Can you work these out from the model? Positions are in its coordinate system, mm. A direction names the side the tool comes from. Round coordinates to 2 decimals unless told otherwise and drop trailing zeros. Order: outer loops, then holes, each group sorted by start corner. A loop starts at its lowest first (then second) coordinate and runs counter-clockwise, first axis right, second up. Notation, with made-up numbers: M 62.5,-3.5 L 98.5,-3.5 A35 ccw 98.5,34.5 Z; hole C -39,21 d3. An arc over 180 degrees is marked long. One line per question, with ' | ' between items.
Autodesk Inventor part; units mm, degrees
ref_plane "Work Plane2" through (30.0013, 0, 7.4992) normal (0, 0, -1) x (-1, 0, 0)
ref_plane "YZ Plane" through (0, 0, 0) normal (1, 0, 0) x (0, 1, 0)
ref_plane "XZ Plane" through (0, 0, 0) normal (0, 1, 0) x (-1, 0, 0)
sketch "Sketch1" plane through (0, 0, 0) normal (0, 1, 0) x (-1, 0, 0)
  line L0 (40, 90) -> (-40, 90)
  line L1 (-40, 90) -> (-40, -81.7795)
  line L2 (40, -41.5685) -> (40, 90)
  line L3 (40, 90) -> (-40, -90) construction
  line L4 (-40, 90) -> (40, -90) construction
  circle A0 centre (-0.0013, 54.9992) radius 5.1
  line L5 (23.4987, -16.5008) -> (-23.5013, -16.5008) construction
  line L6 (-23.5013, -16.5008) -> (-23.5013, -63.5008) construction
  line L7 (-23.5013, -63.5008) -> (23.4987, -63.5008) construction
  line L8 (23.4987, -63.5008) -> (23.4987, -16.5008) construction
  line L9 (23.4987, -16.5008) -> (-23.5013, -63.5008) construction
  line L10 (-23.5013, -16.5008) -> (23.4987, -63.5008) construction
  circle A1 centre (23.4987, -16.5008) radius 2.75
  circle A2 centre (23.4987, -63.5008) radius 2.75
  circle A3 centre (-23.5013, -16.5008) radius 2.75
  circle A4 centre (-23.5013, -63.5008) radius 2.75
  line L11 (-0.0013, -90.0008) -> (-0.0013, -80) construction
  line L12 (19.9987, -11.0008) -> (-20.0013, -11.0008) construction
  line L13 (-20.0013, -11.0008) -> (-20.0013, -69.0008) construction
  line L14 (-20.0013, -69.0008) -> (19.9987, -69.0008) construction
  line L15 (19.9987, -69.0008) -> (19.9987, -11.0008) construction
  line L16 (19.9987, -11.0008) -> (-20.0013, -69.0008) construction
  line L17 (-20.0013, -11.0008) -> (19.9987, -69.0008) construction
  line L18 (-29.0013, -60.0008) -> (28.9987, -60.0008) construction
  line L19 (28.9987, -60.0008) -> (28.9987, -20.0008) construction
  line L20 (28.9987, -20.0008) -> (-29.0013, -20.0008) construction
  line L21 (-29.0013, -20.0008) -> (-29.0013, -60.0008)
  line L22 (-29.0013, -60.0008) -> (28.9987, -20.0008) construction
  line L23 (28.9987, -60.0008) -> (-29.0013, -20.0008) construction
  line L24 (-0.0013, 54.9992) -> (102.5291, -47.5313) construction
  line L25 (-0.0013, 54.9992) -> (144.9987, 54.9992) construction
  line L26 (28.2843, 83.2843) -> (-28.2843, 26.7157) construction
  line L27 (-28.2843, 26.7157) -> (74.2462, -75.8148) construction
  line L28 (74.2462, -75.8148) -> (130.8148, -19.2462) construction
  line L29 (130.8148, -19.2462) -> (28.2843, 83.2843) construction
  line L30 (28.2843, 83.2843) -> (74.2462, -75.8148) construction
  line L31 (-28.2843, 26.7157) -> (130.8148, -19.2462) construction
  line L32 (74.2462, -75.8148) -> (14.1407, -135.9202)
  line L33 (14.1407, -135.9202) -> (-0.0014, -121.7781)
  line L34 (-0.0014, -121.7781) -> (-31.7795, -90)
  line L35 (74.2462, -75.8148) -> (40, -41.5685)
  line L36 (-31.7795, -90) -> (-40, -81.7795)
  line L37 (44.1935, -105.8675) -> (37.1224, -98.7964)
  line L38 (37.1224, -98.7964) -> (52.1488, -83.7701) construction
  line L39 (37.1224, -98.7964) -> (22.096, -113.8228) construction
  circle A5 centre (52.1488, -83.7701) radius 2.75
  circle A6 centre (22.096, -113.8228) radius 2.75
  line L40 (-0.0013, 54.9992) -> (-0.0013, -40.0008)
  circle A7 centre (-0.0013, -40.0008) radius 22.5
  point P0 (0, 0)
  point P1 (51.2639, 3.7339)
  dimension "d0" = 80
  dimension "d1" = 180
  dimension "d3" = 10.2
  dimension "d5" = 47
  dimension "d6" = 47
  dimension "d7" = 5.5
  dimension "d8" = 5.5
  dimension "d9" = 5.5
  dimension "d10" = 5.5
  dimension "d12" = 40
  dimension "d13" = 58
  dimension "d14" = 58
  dimension "d15" = 40
  dimension "d27" = 45
  dimension "d28" = 145
  dimension "d29" = 80
  dimension "d30" = 145
  dimension "d31" = 85.002
  dimension "d32" = 20
  dimension "d33" = 10
  dimension "d35" = 21.2505
  dimension "d36" = 21.2505
  dimension "d37" = 5.5
  dimension "d38" = 5.5
  dimension "d53" = 95
  dimension "d54" = 45
extrude "Plate3" add sketch "Sketch1" along normal blind 6
fillet "Fillet6" radius 5 4 edges at (-40, 3, -41.5685) (-74.2462, 3, -75.8148) (-14.1407, 3, -135.9202) (40, 3, -81.7795)
fillet "Fillet7" radius 40 2 edges at (40, 3, 90) (-40, 3, 90)
sketch "Sketch2" plane through (0, 0, 0) normal (0, -1, 0) x (1, 0, 0)
  circle A0 centre (0.0013, 54.9992) radius 5.1
  line L0 (0.0013, 54.9992) -> (0.0013, -40.0008) construction
  line L1 (0.0013, 7.4992) -> (55.0013, 7.4992) construction
  line L2 (0.0013, 7.4992) -> (-54.9987, 7.4992) construction
  line L3 (-29.9987, 7.4992) -> (30.0013, 7.4992) construction
  line L4 (-29.9987, 4.7492) -> (30.0013, 4.7492)
  line L5 (30.0013, 10.2492) -> (-29.9987, 10.2492)
  arc A1 (-29.9987, 10.2492) -> (-29.9987, 4.7492) centre (-29.9987, 7.4992) ccw
  arc A2 (30.0013, 4.7492) -> (30.0013, 10.2492) centre (30.0013, 7.4992) ccw
  point P0 (0, 0)
  dimension "d43" = 95
  dimension "d44" = 55
  dimension "d45" = 55
  dimension "d46" = 30
  dimension "d47" = 5.5
extrude "Extrusion1" cut sketch "Sketch2" against normal blind 10 contours A1 L5 A2 L4
ref_plane "Work Plane2" through (30.0013, 0, 7.4992) normal (0, 0, -1) x (-1, 0, 0)
equation "\"d39\" = Thickness"
equation "\"BendRadius\" = Thickness"
equation "\"BendReliefWidth\" = Thickness"
equation "\"BendReliefDepth\" = 0.5 * Thickness"
equation "\"CornerReliefSize\" = 4 * Thickness"
equation "\"MinimumRemnant\" = 2 * Thickness"
equation "\"TransitionRadius\" = BendRadius"
equation "\"JacobiRadiusSize\" = BendRadius"
equation "\"GapSize\" = Thickness"
properties part number "NEMA23MountPlatev2" material "Aluminum 6061"
(1) Please list where these lines run through material, in increasing order: probe 1 along Z at (x, y) = (-9, 3.2); probe 2 along Z at (x, y) = (4, 4.05); probe 3 along Z at (x, y) = (23, 2.7). Write a range as [from, to].
Final values:
probe 1: [-130.78, -60.62], [-19.38, 4.75], [10.25, 88.97] | probe 2: [-117.78, -62.14], [-17.86, 4.75], [10.25, 51.83], [58.16, 89.8] | probe 3: [-98.78, -66.2], [-60.8, -19.2], [-13.8, 4.75], [10.25, 82.73]
(2) If we section it at D-D on z = 2: Please give me the cut outline in (x, y).
Final values:
outline: M -40,0 L 40,0 L 40,6 L -40,6 Z
(3) Will these pins go through, and if not, where does the flat tip stop? pin 1 Ø2 at (x, y) = (15.5, 3) entering from +Z; pin 2 Ø2 at (x, y) = (-39, 3) entering from -Z; pin 3 Ø1.8 at (x, y) = (12.5, 1.5) entering from +Z.
Final values:
pin 1: z = 87.28 | pin 2: z = -112.06 | pin 3: z = 88.28
(4) If we section it at B-B on y = 1.6: State how many separate pieces and enclosed holes the cut face has, plus the area to 3 significant figures.
Final values:
separate pieces: 1 | enclosed holes: 9 | area: 14,600 mm^2
(5) Thinking about a two-plate mould opening in X: for faces 1 (the cylindrical face through (4.879, 2.958, -18.036)), 2 (the cylindrical face through (-72.175, 3.042, -75.87)), 3 (the flat face through (13.62, 2.96, -108.16)), which applies, released by +X, released by -X, zero draft, split by the parting line, or undercut?
Final values:
face 1: undercut | face 2: released by -X | face 3: released by +X
(6) On a 3-axis mill with a long thin cutter (end or side, diameter ignored), from which of +Z, -Z, +X, -X, +Y, -Y can I reach the whole of each face in a straight line? I mean faces 4 (the flat face through (0, 3, 4.749)), 5 (the cylindrical face through (27.972, 3.042, 78.594)), 6 (the flat face through (-40, 3, 5)). Say none if no direction works.
Final values:
face 4: +Y, -Y | face 5: +Z, +X, +Y, -Y | face 6: +Z, -X, +Y, -Y
(7) If we section it at A-A on x = 10: Please give me the cut outline in (y, z), plus the area to 3 significant figures.
Final values:
outline: M 0,-111.78 L 6,-111.78 L 6,-60.16 L 0,-60.16 Z; M 0,-19.84 L 6,-19.84 L 6,4.75 L 0,4.75 Z; M 0,10.25 L 6,10.25 L 6,88.73 L 0,88.73 Z | area: 928 mm^2
(8) If we section it at C-C on z = -28: Please give me the cut outline in (x, y).
Final values:
outline: M -40,0 L -19.03,0 L -19.03,6 L -40,6 Z; M 19.03,0 L 40,0 L 40,6 L 19.03,6 Z
